Verification items for the finished model (mm, model axes). Face numbers are marked on the shaded views. A direction names the side the tool comes from. Give positions to 0.01 mm unless a question says otherwise; leave off trailing zeros. Order: outer loops, then holes, each group sorted by start corner. A loop starts at its lowest first (then second) coordinate and runs counter-clockwise, first axis right, second up. Notation, with made-up numbers: (53, -15) -> (73, -15) arc R36 ccw to (73, 23) -> close; hole circle Ø10 at (10.25, -14). An arc over 180 degrees is marked (long way). Return JSON: item names as keys, results as strings. Group by question number.
(1) Cross-section at B-B on z = 0. Enter the section's corners in (x, y).
(2) Cross-section at A-A on x = -26.45. Enter the section's corners in (y, z).
(3) Cross-section at D-D on z = 4. State how many separate pieces and enclosed holes the cut face has, then the cut area to 3 significant figures.
(4) Tool access check on the marked faces 4, 5 and 6. Record the directions out of +Z, -Z, +X, -X, +Y, -Y that give a thin tool (end or side, any length) a straight path to the whole face; none if there is none.
(5) Cross-section at C-C on x = -12.5. Enter the section's corners in (y, z).
(6) Release check for a two-part mould opening along X. For the marked faces 1, 2 and 3 record: pulls with the +X half, pulls with the -X half, needs draft (parallel to the pull), parting line crosses it, or undercut.
(7) Thickness scan on line 1 along Z through (x, y) = (26.45, 10.6); line 2 along Z through (x, y) = (-26.45, 10.9); line 3 along X through (y, z) = (11.45, -5). Record the ranges inside material, lowest first.
(8) Depth check by flat-ended pin: pin 1 Ø6.5 at (x, z) = (26.45, 5.15) entering from -Y; pin 2 Ø4 at (y, z) = (2, 4) entering from +X; pin 3 Ø5.5 at (x, z) = (21, 4) entering from -Y. Enter the tip coordinate at first touch or a pass-through.
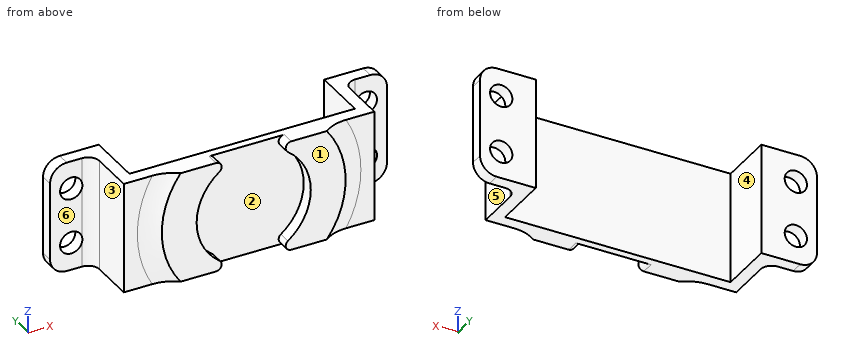
from build123d import *

# Parameters (mm, degrees)
SKETCH1_W           = 45
SKETCH1_H           = 20
BOSS_EXTRUDE1_DEPTH = 2.25
SKETCH2_W           = 2.25
SKETCH2_H           = 20
BOSS_EXTRUDE2_DEPTH = 10
SKETCH3_W           = 10
SKETCH3_H           = 20
BOSS_EXTRUDE3_DEPTH = 2.3
FILLET1_R           = 2
SKETCH4_R           = 2
CUT_EXTRUDE1_DEPTH  = 35.133927404
BOSS_EXTRUDE5_DEPTH = 1.5
SKETCH6_R           = 10.25
CUT_EXTRUDE2_DEPTH  = 2.3
FILLET2_R           = 5
FILLET3_R           = 1
FILLET4_R           = 3


with BuildPart() as part:
    # Sketch1 → Boss-Extrude1 (new body)
    with BuildSketch(Plane(origin=(0, 0, 0), x_dir=(1, 0, 0), z_dir=(0, 1, 0))):
        Rectangle(SKETCH1_W, SKETCH1_H)
    extrude(amount=BOSS_EXTRUDE1_DEPTH)

    # Sketch2 → Boss-Extrude2 (add)
    with BuildSketch(Plane(origin=(0, 2.25, 0), x_dir=(1, 0, 0), z_dir=(0, 1, 0))):
        with Locations((-21.375, 0)):
            Rectangle(SKETCH2_W, SKETCH2_H)
        with Locations((21.375, 0)):
            Rectangle(SKETCH2_W, SKETCH2_H)
    extrude(amount=BOSS_EXTRUDE2_DEPTH)

    # Sketch3 → Boss-Extrude3 (add)
    with BuildSketch(Plane(origin=(0, 12.25, 0), x_dir=(1, 0, 0), z_dir=(0, 1, 0))):
        with Locations((-25.25, 0)):
            Rectangle(SKETCH3_W, SKETCH3_H)
        with Locations((25.25, 0)):
            Rectangle(SKETCH3_W, SKETCH3_H)
    extrude(amount=-BOSS_EXTRUDE3_DEPTH)

    # Fillet1
    fillet1_edges = [part.edges().sort_by_distance(p)[0] for p in [
        (-22.5, 9.95, 0),
        (22.5, 9.95, 0),
    ]]
    fillet(fillet1_edges, radius=FILLET1_R)

    # Sketch4 → Cut-Extrude1 (cut, through all)
    with BuildSketch(Plane(origin=(0, 12.25, 0), x_dir=(1, 0, 0), z_dir=(0, 1, 0))):
        with Locations(Location((26.45, 5.15278214, 0), (0, 0, 270))):
            Circle(SKETCH4_R)
        with Locations(Location((26.45, -5.15278214, 0), (0, 0, 270))):
            Circle(SKETCH4_R)
        with Locations(Location((-26.45, 5, 0), (0, 0, 270))):
            Circle(SKETCH4_R)
        with Locations(Location((-26.45, -5, 0), (0, 0, 270))):
            Circle(SKETCH4_R)
    extrude(amount=-CUT_EXTRUDE1_DEPTH, mode=Mode.SUBTRACT)

    # Sketch5 → Boss-Extrude5 (add)
    with BuildSketch(Plane.XZ):
        with BuildLine():
            Line((13.124404748, 10), (-13.124404748, 10))
            ThreePointArc((-13.124404748, 10), (-16.5, 0), (-13.124404748, -10))
            Line((-13.124404748, -10), (13.124404748, -10))
            ThreePointArc((13.124404748, -10), (16.5, 0), (13.124404748, 10))
        make_face()
    extrude(amount=BOSS_EXTRUDE5_DEPTH)

    # Sketch6 → Cut-Extrude2 (cut)
    with BuildSketch(Plane.XZ.offset(1.5)):
        Circle(SKETCH6_R)
    extrude(amount=-CUT_EXTRUDE2_DEPTH, mode=Mode.SUBTRACT)

    # Fillet2
    # the kernel refuses this fillet: 5 mm, written as the material it adds along each edge
    with BuildSketch(Plane(origin=(0, 0, 0), x_dir=(0.3695559443518841, 0, -0.9292084825238021), z_dir=(-0.9292084825238021, 0, -0.3695559443518841))) as fillet2_piece_1_section:
        with BuildLine():
            CenterArc((20.070714214, 5), FILLET2_R, 224.427004001, 45.572995999)
            Line((16.5, 1.5), (16.428585716, 1.43))
            ThreePointArc((16.428585716, 1.43), (16.4, 0.75), (16.4, 0))
            Line((16.4, 0), (16.5, -0.1))
            Line((16.5, -0.1), (20.070714214, -0.1))
            Line((20.070714214, -0.1), (20.070714214, 0))
        make_face()
    fillet2_piece_1 = revolve(axis=Axis((0, 0, 0), (0, -1, 0)), revolution_arc=136.623532333, mode=Mode.PRIVATE)
    fillet2_piece_1 = split(fillet2_piece_1, bisect_by=Plane(origin=(18.120334402, -0.357167387, 10), z_dir=(0, 0, -1)), keep=Keep.TOP, mode=Mode.PRIVATE)
    fillet2_piece_1 = split(fillet2_piece_1, bisect_by=Plane(origin=(18.120334402, -0.357167387, -10), z_dir=(0, 0, 1)), keep=Keep.TOP, mode=Mode.PRIVATE)
    add(fillet2_piece_1)
    with BuildSketch(Plane(origin=(0, 0, 0), x_dir=(-0.3695559443518876, 0, 0.9292084825238008), z_dir=(0.9292084825238008, 0, 0.3695559443518876))) as fillet2_piece_2_section:
        with BuildLine():
            CenterArc((20.070714214, 5), FILLET2_R, 224.427004001, 45.572995999)
            Line((20.070714214, 0), (20.070714214, -0.1))
            Line((20.070714214, -0.1), (16.5, -0.1))
            Line((16.5, -0.1), (16.4, 0))
            ThreePointArc((16.4, 0), (16.4, 0.75), (16.428585716, 1.43))
            Line((16.428585716, 1.43), (16.5, 1.5))
        make_face()
    fillet2_piece_2 = revolve(axis=Axis((0, 0, 0), (0, -1, 0)), revolution_arc=136.623532333, mode=Mode.PRIVATE)
    fillet2_piece_2 = split(fillet2_piece_2, bisect_by=Plane(origin=(-18.120334402, -0.357167387, 10), z_dir=(0, 0, -1)), keep=Keep.TOP, mode=Mode.PRIVATE)
    fillet2_piece_2 = split(fillet2_piece_2, bisect_by=Plane(origin=(-18.120334402, -0.357167387, -10), z_dir=(0, 0, 1)), keep=Keep.TOP, mode=Mode.PRIVATE)
    add(fillet2_piece_2)

    # Fillet3
    fillet3_edges = [part.edges().sort_by_distance(p)[0] for p in [
        (-2.25, -0.35, -10),
        (-2.25, -0.35, 10),
        (2.25, -0.35, -10),
        (2.25, -0.35, 10),
    ]]
    fillet(fillet3_edges, radius=FILLET3_R)

    # Fillet4
    fillet4_edges = [part.edges().sort_by_distance(p)[0] for p in [
        (-30.25, 11.1, -10),
        (-30.25, 11.1, 10),
        (30.25, 11.1, 10),
        (30.25, 11.1, -10),
    ]]
    fillet(fillet4_edges, radius=FILLET4_R)


solid = part.part
Verdict:
{
 "1": {"outline": "(-30.25, 9.95) -> (-24.5, 9.95) arc R2 cw to (-22.5, 7.95) -> (-22.5, 0) -> (-20.07, 0) arc R5 cw to (-16.5, -1.5) -> (-10.25, -1.5) -> (-10.25, 0.8) -> (10.25, 0.8) -> (10.25, -1.5) -> (16.5, -1.5) arc R5 cw to (20.07, 0) -> (22.5, 0) -> (22.5, 7.95) arc R2 cw to (24.5, 9.95) -> (30.25, 9.95) -> (30.25, 12.25) -> (20.25, 12.25) -> (20.25, 2.25) -> (-20.25, 2.25) -> (-20.25, 12.25) -> (-30.25, 12.25) -> close"},
 "2": {"outline": "(9.95, -10) -> (12.25, -10) -> (12.25, -7) -> (9.95, -7) -> close; (9.95, -3) -> (12.25, -3) -> (12.25, 3) -> (9.95, 3) -> close; (9.95, 7) -> (12.25, 7) -> (12.25, 10) -> (9.95, 10) -> close"},
 "3": {"separate pieces": "3", "enclosed holes": "0", "area": "176 mm²"},
 "4": {"face 4": "+Z, -Z, +Y", "face 5": "+Z, -Z, +X, -Y", "face 6": "+Z, -Z, -X, -Y"},
 "5": {"outline": "(-1.5, -10) -> (2.25, -10) -> (2.25, 10) -> (-1.5, 10) -> close"},
 "6": {"face 1": "needs draft", "face 2": "undercut", "face 3": "pulls with the -X half"},
 "7": {"line 1": "-10 to -7.15, -3.15 to 3.15, 7.15 to 10", "line 2": "-10 to -7, -3 to 3, 7 to 10", "line 3": "-30.25 to -28.45, -24.45 to -20.25, 20.25 to 24.46, 28.44 to 30.25"},
 "8": {"pin 1": "y = 9.47", "pin 2": "x = 22.5", "pin 3": "y = -0.21"}
}
